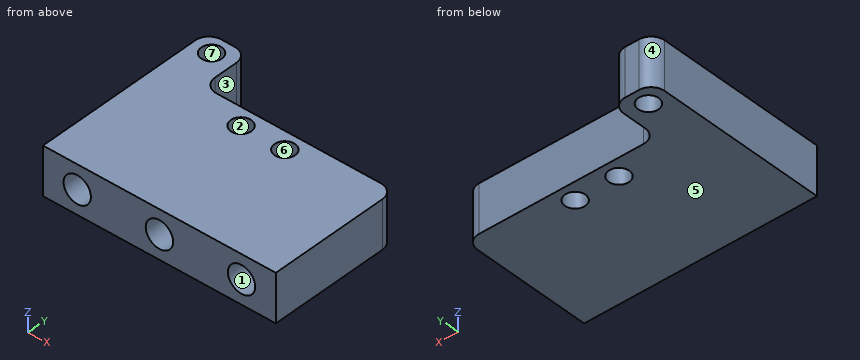
Autodesk Inventor part; units mm, degrees
ref_plane "YZ Plane" through (0, 0, 0) normal (1, 0, 0) x (0, 1, 0)
ref_plane "XZ Plane" through (0, 0, 0) normal (0, 1, 0) x (-1, 0, 0)
ref_plane "XY Plane" through (0, 0, 0) normal (0, 0, 1) x (1, 0, 0)
sketch "Sketch1" plane through (0, 0, 0) normal (0, 1, 0) x (-1, 0, 0)
  circle A0 centre (0, 0) radius 2
  circle A1 centre (12, 0) radius 2
  line L0 (0, 0) -> (0, 2) construction
  circle A2 centre (-12, 0) radius 2
  line L1 (17, 3.5) -> (-17, 3.5)
  line L2 (-17, 3.5) -> (-17, -3.5)
  line L3 (-17, -3.5) -> (17, -3.5)
  line L4 (17, -3.5) -> (17, 3.5)
  line L5 (17, 3.5) -> (-17, -3.5) construction
  line L6 (-17, 3.5) -> (17, -3.5) construction
  dimension "d0" = 4
  dimension "d1" = 4
  dimension "d2" = 12
  dimension "d3" = 34
  dimension "d4" = 7
extrude "Extrusion1" add sketch "Sketch1" along normal blind 27 contours A0 | A1 | A2 | L4 L3 L2 L1
extrude "Extrusion2" cut sketch "Sketch1" along normal blind 8 contours A0 | A1 | A2
sketch "Sketch2" plane through (-17, 0, 3.5) normal (0, 0, 1) x (1, 0, 0)
  circle A0 centre (20.2, 17) radius 1.5
  circle A1 centre (13.8, 17) radius 1.5
  circle A2 centre (2.825, 24.5) radius 1.5
  line L0 (13.8, 17) -> (20.2, 17) construction
  line L1 (0, 0) -> (34, 0)
  line L2 (0, 27) -> (34, 27) construction
  point P0 (17, 0)
  point P1 (17, 17)
  point P2 (17, 0)
  point P3 (17, 27)
  dimension "d9" = 3
  dimension "d10" = 3
  dimension "d11" = 3
  dimension "d12" = 6.4
  dimension "d13" = 10.975
  dimension "d14" = 7.5
  dimension "d15" = 10
extrude "Extrusion3" cut sketch "Sketch2" against normal through all
sketch "Sketch3" plane through (-17, 0, 3.5) normal (0, 0, 1) x (1, 0, 0)
  line L0 (34, 27) -> (0, 27)
  line L1 (6, 27) -> (6, 19.5)
  line L2 (6, 19.5) -> (34, 19.5)
  line L3 (34, 0) -> (34, 27)
  point P0 (17, 0)
  dimension "d18" = 7.5
  dimension "d19" = 28
extrude "Extrusion4" cut sketch "Sketch3" against normal through all
fillet "Fillet1" radius 2 4 edges at (-17, 27, 0) (-11, 27, 0) (-11, 19.5, 0) (17, 19.5, 0)
properties part number "Pixy2Mount" material "PC/ABS Plastic"
Work out the finished part from the listing and answer in its coordinate system (mm). Face numbers are marked on the shaded views. A direction names the side the tool comes from. Round coordinates to 2 decimals unless told otherwise and drop trailing zeros. Write each loop counter-clockwise with the first axis right and the second up, starting at its lowest first coordinate (ties: lowest second). Pieces come first, ordered by that corner, then holes. Notation, with made-up numbers: (88.25, -28) - (97.25, -28) arc R12 ccw to (97.25, -14) - close; hole circle Ø11 at (-27, -38). An arc over 180 degrees is marked (long way). Return JSON: item names as keys, results as strings. Group by question number.
Q1. The part is cut by section D-D on z = -3. Write down the section's boundary in (x, y) (3 decimals), then the cut area to 3 significant figures.
Q2. The part is cut by section A-A on y = 17. Write down the section's boundary in (x, z).
Q3. The part is cut by section B-B on y = 3.75. Write down the section's boundary in (x, z).
Q4. Find the intervals of material crossed by L1, parallel to X at y = 4.5, z = -1.5; L2, parallel to Z at x = -12, y = 6.75; L3, parallel to X at y = 16.25, z = 0, in increasing order.
Q5. For the marked faces 1, 2 and 3, determine the directions among +Z, -Z, +X, -X, +Y, -Y from which every point of the face is accessible in a straight line to the end or side of a thin tool.
Q6. The mould has two halves that part along Y. Classify the marked faces 4, 5, 6 and 7: released by +Y, released by -Y, zero draft, split by the parting line, or undercut.
Q7. The part is cut by section C-C on x = 3.2. Write down the section's boundary in (y, z), then the cut area to 4 significant figures.
Q8. Each of these flat-tipped pins is pushed along its axis until it touches: pin 1 Ø4 at (y, z) = (23.5, 0.5) entering from +X; pin 2 Ø2.5 at (x, y) = (3.2, 17) entering from +Z; pin 3 Ø2 at (x, z) = (7.5, 1) entering from +Y. Where does it stop, or does it pass through?
Solved:
{
 "1": {"outline": "(-17, 0) - (17, 0) - (17, 17.5) arc R2 ccw to (15, 19.5) - (-9, 19.5) arc R2 cw to (-11, 21.5) - (-11, 25) arc R2 ccw to (-13, 27) - (-15, 27) arc R2 ccw to (-17, 25) - close; hole circle Ø3 at (-14.175, 24.5); hole circle Ø3 at (-3.2, 17); hole circle Ø3 at (3.2, 17)", "area": "685 mm²"},
 "2": {"outline": "(-17, -3.5) - (-4.7, -3.5) - (-4.7, 3.5) - (-17, 3.5) - close; (-1.7, -3.5) - (1.7, -3.5) - (1.7, 3.5) - (-1.7, 3.5) - close; (4.7, -3.5) - (17, -3.5) - (17, 3.5) - (4.7, 3.5) - close"},
 "3": {"outline": "(-17, -3.5) - (17, -3.5) - (17, 3.5) - (-17, 3.5) - close; hole circle Ø4 at (-12, 0); hole circle Ø4 at (0, 0); hole circle Ø4 at (12, 0)"},
 "4": {"L1": "-17 to -13.32, -10.68 to -1.32, 1.32 to 10.68, 13.32 to 17", "L2": "-3.5 to -2, 2 to 3.5", "L3": "-17 to -4.5, -1.9 to 1.9, 4.5 to 17"},
 "5": {"face 1": "-Y", "face 2": "+Z, -Z", "face 3": "+Z, -Z, +X, +Y"},
 "6": {"face 4": "released by +Y", "face 5": "zero draft", "face 6": "undercut", "face 7": "undercut"},
 "7": {"outline": "(0, -3.5) - (15.5, -3.5) - (15.5, 3.5) - (0, 3.5) - close; (18.5, -3.5) - (19.5, -3.5) - (19.5, 3.5) - (18.5, 3.5) - close", "area": "115.5 mm²"},
 "8": {"pin 1": "x = -11", "pin 2": "through", "pin 3": "y = 19.5"}
}
